```python
from build123d import *

# Parameters (mm, degrees)
BOSS_EXTRUDE1_DEPTH = 10
SKETCH2_R           = 3.95
BOSS_EXTRUDE2_DEPTH = 10
BOSS_EXTRUDE3_DEPTH = 10
SKETCH5_W           = 10
SKETCH5_H           = 60
BOSS_EXTRUDE4_DEPTH = 3
FILLET1_R           = 1
FILLET2_R           = 2
SKETCH7_R           = 1.5
CUT_EXTRUDE1_DEPTH  = 3


with BuildPart() as part:
    # Sketch1 → Boss-Extrude1 (new body)
    with BuildSketch(Plane(origin=(0, 0, 0), x_dir=(0, 0, -1), z_dir=(1, 0, 0))):
        with BuildLine():
            Line((-15, 0), (15, 0))
            Line((15, 0), (9.520917343, 17.058125725))
            ThreePointArc((9.520917343, 17.058125725), (0, 24), (-9.520917343, 17.058125725))
            Line((-9.520917343, 17.058125725), (-15, 0))
        make_face()
    extrude(amount=BOSS_EXTRUDE1_DEPTH)

    # Sketch2 → Boss-Extrude2 (add)
    with BuildSketch(Plane(origin=(10, 0, 0), x_dir=(0, 0, -1), z_dir=(1, 0, 0))):
        with Locations((0, 14)):
            Circle(SKETCH2_R)
    extrude(amount=BOSS_EXTRUDE2_DEPTH)

    # Sketch4 → Boss-Extrude3 (add)
    with BuildSketch(Plane(origin=(10, 0, 0), x_dir=(0, 0, -1), z_dir=(1, 0, 0))):
        with BuildLine():
            Line((9.520917343, 17.058125725), (15, 0))
            Line((15, 0), (13.966745843, 14.964370546))
            ThreePointArc((13.966745843, 14.964370546), (0, 28), (-13.966745843, 14.964370546))
            Line((-13.966745843, 14.964370546), (-15, 0))
            Line((-15, 0), (-9.520917343, 17.058125725))
            ThreePointArc((-9.520917343, 17.058125725), (0, 24), (9.520917343, 17.058125725))
        make_face()
    extrude(amount=-BOSS_EXTRUDE3_DEPTH)

    # Sketch5 → Boss-Extrude4 (add)
    with BuildSketch(Plane.XZ):
        with Locations((5, 0)):
            Rectangle(SKETCH5_W, SKETCH5_H)
    extrude(amount=-BOSS_EXTRUDE4_DEPTH)

    # Fillet1
    fillet1_edges = [part.edges().sort_by_distance(p)[0] for p in [
        (10, 1.5, 30),
        (0, 1.5, -30),
        (0, 1.5, 30),
        (10, 1.5, -30),
    ]]
    fillet(fillet1_edges, radius=FILLET1_R)

    # Fillet2
    fillet2_edges = [part.edges().sort_by_distance(p)[0] for p in [
        (5, 3, -14.792857143),
        (5, 3, 14.792857143),
    ]]
    fillet(fillet2_edges, radius=FILLET2_R)

    # Sketch7 → Cut-Extrude1 (cut)
    with BuildSketch(Plane(origin=(0, 3, 0), x_dir=(1, 0, 0), z_dir=(0, 1, 0))):
        with Locations((5, 22.829761905)):
            Circle(SKETCH7_R)
        with Locations((5, -22.829761905)):
            Circle(SKETCH7_R)
    extrude(amount=-CUT_EXTRUDE1_DEPTH, mode=Mode.SUBTRACT)


solid = part.part
```
Can you work these out from the model? Positions are in its coordinate system, mm. A direction names the side the tool comes from. Coordinates: 2 decimals unless noted, no trailing zeros. Order: outer loops, then holes, each group sorted by start corner. A loop starts at its lowest first (then second) coordinate and runs counter-clockwise, first axis right, second up.
1. If we section it at D-D (y = 17): Please give me the cut outline in (x, z), then the cut area to 3 significant figures.
2. For faces 4 (the face through (5, 3, 25)), 5 (the face through (5, 28, 0)), 6 (the face through (5, 0, 0)), 7 (the face through (14.93, 10.144, 0.856)), 8 (the face through (5, 3, -25)), which set-ups out of +Z, -Z, +X, -X, +Y, -Y let a thin tool reach every point of the face, with its end or its side?
3. I'm going to push flat-ended pins straight in: pin 1 (8 mm diameter, centred on x = 7.5, z = 20, fed in from +Y); pin 2 (8 mm diameter, centred on x = 18, z = -9.5, fed in from +Y); pin 3 (6 mm diameter, centred on y = 4, z = -5.5, fed in from +X); pin 4 (12 mm diameter, centred on x = 6, z = 11.5, fed in from +Y). Where does each tip first touch, or does it pass through?
4. Thinking about a two-plate mould opening in X: for faces 1 (the face through (10, 8, 0)), 2 (the face through (5.07, 3.524, 15.31)), 3 (the face through (4.675, 1.521, -21.365)), which applies, +X half, -X half, draft (parallel to the pull), parting line (faces both ways), or undercut?
5. If we section it at B-B (z = 0): Please give me the cut outline in (x, y), then the cut area to 3 significant figures.
6. I need wall thicknesses on line 1 (Z direction, x = 5, y = 1.65); line 2 (X direction, y = 24, z = -7); line 3 (Y direction, x = 2.75, z = 27). Which ranges of each line are inside material? Lowest first, please.
7. If we section it at C-C (x = 2.25): Please give me the cut outline in (y, z), then the cut area to 3 significant figures.
8. If we section it at A-A (x = 5.75): Please give me the cut outline in (y, z).
Entries:
1. outline: (0, -13.67) - (10, -13.67) - (10, -2.57) - (20, -2.57) - (20, 2.57) - (10, 2.57) - (10, 13.67) - (0, 13.67) - close
1. area: 325 mm2
2. face 4: +Z, +X, -X, +Y
2. face 5: +X, -X, +Y
2. face 6: +Z, -Z, +X, -X, -Y
2. face 7: +X
2. face 8: -Z, +X, -X, +Y
3. pin 1: stops at y = 3.11
3. pin 2: passes through
3. pin 3: stops at x = 10
3. pin 4: stops at y = 26.87
4. face 1: +X half
4. face 2: draft
4. face 3: undercut
5. outline: (0, 0) - (10, 0) - (10, 10.05) - (20, 10.05) - (20, 17.95) - (10, 17.95) - (10, 28) - (0, 28) - close
5. area: 359 mm2
6. line 1: z = -30 to -24.33, -21.33 to 21.33, 24.33 to 30
6. line 2: x = 0 to 10
6. line 3: y = 0 to 3
7. outline: (0, -30) - (3, -30) - (3, -16.66) arc R2 cw to (4.86, -14.66) - (14.96, -13.97) arc R14 ccw to (14.96, 13.97) - (4.86, 14.66) arc R2 cw to (3, 16.66) - (3, 30) - (0, 30) - close
7. area: 806 mm2
8. outline: (0, -30) - (3, -30) - (3, -24.13) - (0, -24.13) - close; (0, -21.53) - (3, -21.53) - (3, -16.66) arc R2 cw to (4.86, -14.66) - (14.96, -13.97) arc R14 ccw to (14.96, 13.97) - (4.86, 14.66) arc R2 cw to (3, 16.66) - (3, 21.53) - (0, 21.53) - close; (0, 24.13) - (3, 24.13) - (3, 30) - (0, 30) - close
